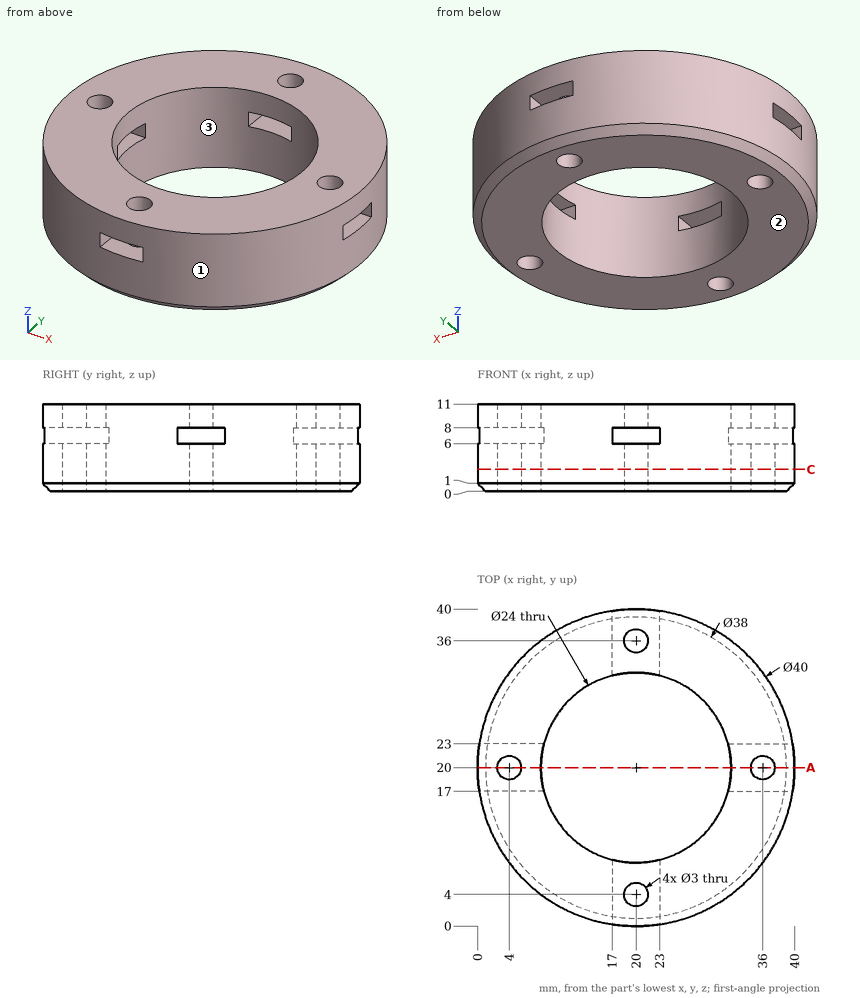
Geometry check sheet. Reference: drawing and pictorial views, mm from the part's lowest x, y, z. Give positions to 0.01 mm unless a question says otherwise; leave off trailing zeros. Order: outer loops, then holes, each group sorted by start corner. A loop starts at its lowest first (then second) coordinate and runs counter-clockwise, first axis right, second up. Notation, with made-up numbers: M -32.75,53.25 L -8.75,53.25 A26 cw -8.75,70.25 Z; hole C 14,5.25 d7. An arc over 180 degrees is marked long. Return JSON: item names as keys, results as strings. Group by question number.
1) Section check C-C on z = 2.75. Record the cut outline in (x, y), and give its area (3 significant figures).
2) Mould release check, pull along X, two halves, no side actions. Record for the marked faces 1, 2 and 3: pulls with the +X half, pulls with the -X half, needs draft (parallel to the pull), parting line crosses it, or undercut.
3) Scan lines: line 1 (X direction, y = 20, z = 2.55); line 2 (Z direction, x = 18.5, y = 3). Record each from-to range of solid material in increasing order.
4) Section check A-A on y = 20. Give the number of separate pieces and of enclosed holes in the cut face, and give its area (3 significant figures).
5) Go/stop test with flat-tipped pins: pin 1 Ø2 at (y, z) = (35.5, 7) entering from +X (3 decimals); pin 2 Ø2 at (x, z) = (15, 7) entering from +Y; pin 3 Ø3 at (x, z) = (29, 6) entering from +Y. Record where each tip stops, or that it passes through.
Answer block:
{
 "1": {"outline": "C 20,20 d40; hole C 4,20 d3; hole C 20,20 d24; hole C 20,4 d3; hole C 20,36 d3; hole C 36,20 d3", "area": "776 mm^2"},
 "2": {"face 1": "parting line crosses it", "face 2": "needs draft", "face 3": "undercut"},
 "3": {"line 1": "x = 0 to 2.5, 5.5 to 8, 32 to 34.5, 37.5 to 40", "line 2": "z = 0 to 6, 8 to 11"},
 "4": {"separate pieces": "8", "enclosed holes": "0", "area": "89.0 mm^2"},
 "5": {"pin 1": "stops at x = 33.775", "pin 2": "stops at y = 39.6", "pin 3": "stops at y = 38.54"}
}
